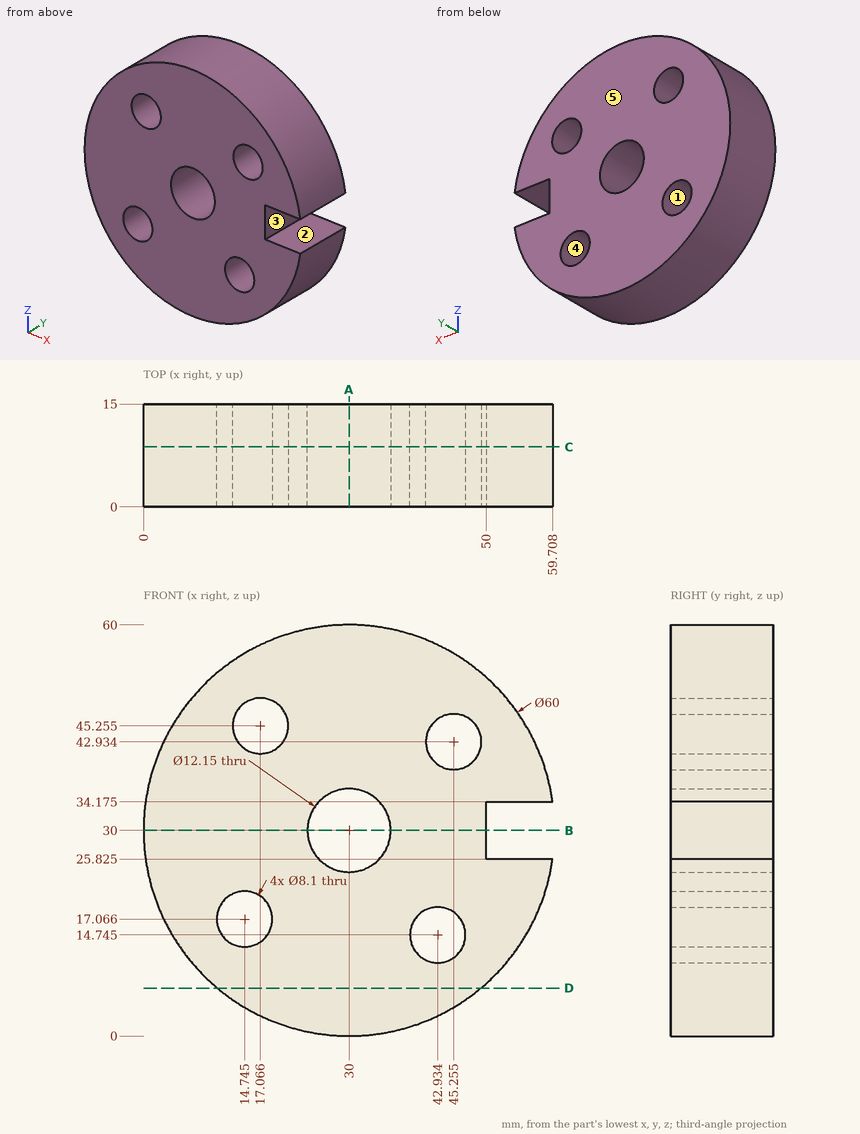
The figure shows three views and two pictorial views of one solid part (mm, origin at its lowest corner). Answer the questions. A direction names the side the tool comes from. Coordinates: 2 decimals unless noted, no trailing zeros. Loops run counter-clockwise (first coordinate to the right, second up) from the corner with the lowest first, then second, coordinate; pieces in that order, holes last.
1) Determine the mould class of the marked faces 3, 4 and 5 for opening direction X: pulls with the +X half, pulls with the -X half, needs draft (parallel to the pull), parting line crosses it, or undercut.
2) Find the intervals of material crossed by L1, parallel to X at y = 5.75, z = 30 (1 decimal); L2, parallel to X at y = 2.75, z = 13.5 (1 decimal); L3, parallel to X at y = 4, z = 25, in increasing order.
3) Flat-ended cylindrical pins translate along their axes: pin 1 Ø2.5 at (y, z) = (5.5, 29) entering from +X; pin 2 Ø7.5 at (x, z) = (42.93, 14.74) entering from +Y; pin 3 Ø3 at (x, y) = (56, 10) entering from +Z (1 decimal); pin 4 Ø5 at (x, y) = (21.5, 6) entering from -Z. Find the tip coordinate at first contact, or state that the pin passes through.
4) Find section A-A on x = 30. Write down the section's boundary in (y, z) (1 decimal), then the cut area to 3 significant figures.
5) Find section D-D on z = 7. Write down the section's boundary in (x, y).
6) A tool of negligible diameter and unlimited length cuts with its end or side. For the marked faces 1 and 2, from which of +Z, -Z, +X, -X, +Y, -Y can it reach the whole face along a straight path? Write none if from no direction.
7) Find section B-B on z = 30. Write down the section's boundary in (x, y) (1 decimal).
8) Find section C-C on y = 8.75. Give the number of separate pieces and of enclosed holes in the cut face, then the cut area to 3 significant figures.
Values:
1. face 3: pulls with the +X half
1. face 4: undercut
1. face 5: needs draft
2. L1: x = 0 to 23.9, 36.1 to 50
2. L2: x = 4.9 to 12.8, 16.7 to 39.1, 46.8 to 55.1
2. L3: x = 0.42 to 26.55, 33.45 to 59.58
3. pin 1: stops at x = 50
3. pin 2: passes through
3. pin 3: stops at z = 47.3
3. pin 4: stops at z = 0.61
4. outline: (0, 0) - (15, 0) - (15, 23.9) - (0, 23.9) - close; (0, 36.1) - (15, 36.1) - (15, 60) - (0, 60) - close
4. area: 718 mm2
5. outline: (10.74, 0) - (49.26, 0) - (49.26, 15) - (10.74, 15) - close
6. face 1: +Y, -Y
6. face 2: +X, +Y, -Y
7. outline: (0, 0) - (23.9, 0) - (23.9, 15) - (0, 15) - close; (36.1, 0) - (50, 0) - (50, 15) - (36.1, 15) - close
8. separate pieces: 1
8. enclosed holes: 5
8. area: 2,420 mm2
